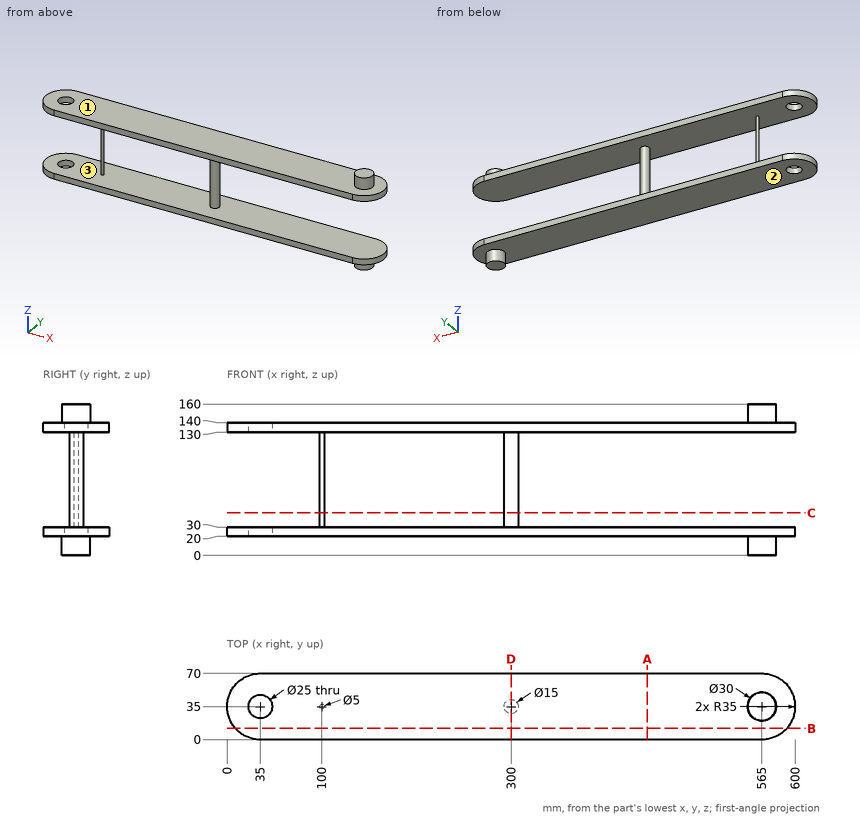
Verification items for this drawing (mm, ordinates from the low corner). Coordinates: 2 decimals unless noted, no trailing zeros. Write each loop counter-clockwise with the first axis right and the second up, starting at its lowest first coordinate (ties: lowest second). Pieces come first, ordered by that corner, then holes. Notation, with made-up numbers: (72.25, 39) - (92.25, 39) arc R20 cw to (92.25, 77) - close; hole circle Ø3 at (7, 25). An arc over 180 degrees is marked (long way). One line per question, with ' | ' between items.
Item 1: Mould release check, pull along Z, two halves, no side actions. Record for the marked faces 1, 2 and 3: pulls with the +Z half, pulls with the -Z half, needs draft (parallel to the pull), parting line crosses it, or undercut.
Determined:
face 1: pulls with the +Z half | face 2: pulls with the -Z half | face 3: undercut
Item 2: Thickness scan on line 1 (Y direction, x = 35, z = 136); line 2 (Z direction, x = 370, y = 53); line 3 (Z direction, x = 558, y = 29.5). Record the ranges inside material, lowest first. Write a range as [from, to].
Determined:
line 1: y = [0, 22.5], [47.5, 70] | line 2: z = [20, 30], [130, 140] | line 3: z = [0, 30], [130, 160]
Item 3: Sectioned sample at B-B on y = 12. Record the boundary of the cut face in (x, z), plus the area to 3 significant figures.
Determined:
outline: (8.62, 20) - (591.38, 20) - (591.38, 30) - (8.62, 30) - close; (8.62, 130) - (591.38, 130) - (591.38, 140) - (8.62, 140) - close | area: 11,700 mm2
Item 4: Sectioned sample at A-A on x = 444. Record the boundary of the cut face in (y, z).
Determined:
outline: (0, 20) - (70, 20) - (70, 30) - (0, 30) - close; (0, 130) - (70, 130) - (70, 140) - (0, 140) - close
Item 5: Gauge pin test, flat ends, axial feed: P1, Ø21, axis at x = 411.5, y = 35, coming from the +Z side; P2, Ø6, axis at x = 235, y = 11.5, coming from the -Z side; P3, Ø6, axis at y = 26, z = 25.5, coming from the +X side. Record the tip position at first contact, or that the pin passes through.
Determined:
P1: stops at z = 140 | P2: stops at z = 20 | P3: stops at x = 599.48
Item 6: Sectioned sample at C-C on z = 45. Record the boundary of the cut face in (x, y), plus the area to 3 significant figures.
Determined:
outline: circle Ø5 at (100, 35); circle Ø15 at (300, 35) | area: 196 mm2
Item 7: Sectioned sample at D-D on x = 300. Record the boundary of the cut face in (y, z), plus the area to 3 significant figures.
Determined:
outline: (0, 20) - (70, 20) - (70, 30) - (42.5, 30) - (42.5, 130) - (70, 130) - (70, 140) - (0, 140) - (0, 130) - (27.5, 130) - (27.5, 30) - (0, 30) - close | area: 2,900 mm2
